The model under review builds one solid part; all positions refer to its coordinate system, in mm. Face numbers are marked on the shaded views. A direction names the side the tool comes from. Give positions to 0.01 mm unless a question says otherwise; leave off trailing zeros. Order: outer loops, then holes, each group sorted by start corner. A loop starts at its lowest first (then second) coordinate and runs counter-clockwise, first axis right, second up. Notation, with made-up numbers: (49, 14.5) - (108, 14.5) arc R29 cw to (108, 51.5) - close; hole circle Ø8 at (12, 40). An arc over 180 degrees is marked (long way). Write item = value, one per line. Start each with the question number.
1. We need section B-B, the plane x = -41.5. Give the boundary of the cut face in (y, z), and give its area (3 significant figures).
2. Wall thickness on probe 1 along Z at (x, y) = (48, -22.5); probe 2 along X at (y, z) = (-19.5, 55); probe 3 along Y at (x, z) = (-24, 51): over which ranges is each line inside the solid? List them lowest first.
3. We need section D-D, the plane x = -1. Give the boundary of the cut face in (y, z), and give its area (3 significant figures).
4. Mouldability with a two-part tool opening along Z and no side actions: class the marked faces 5, 6 and 7 as pulls with the +Z half, pulls with the -Z half, needs draft (parallel to the pull), parting line crosses it, or undercut.
5. For P1, Ø10.5, axis at x = -7, y = -28, coming from the +Z side; P2, Ø4, axis at x = 25, y = 34, coming from the +Z side; P3, Ø12, axis at y = -14.5, z = 24.5, coming from the +X side; P4, Ø8, axis at x = 15.5, z = 73, coming from the -Y side, all flat-tipped, find the tip position at first contact; note any pin that passes through.
6. We need section A-A, the plane y = 0. Give the boundary of the cut face in (x, z).
7. Machinability: for the marked faces 1, 2, 3 and 4, which of the approach directions +Z, -Z, +X, -X, +Y, -Y give a long, thin tool a straight path to every point of the face, cutting with its end or side? Answer none if there is none.
8. We need section C-C, the plane y = 21. Give the boundary of the cut face in (x, z), and give its area (3 significant figures).
from build123d import *

# Parameters (mm, degrees)
F0_W     = 101.6
F0_H     = 48.768
F1_DEPTH = 56.388
F0_H_2   = 13.335
F2_DEPTH = 2.54
F3_R     = 4.7625
F4_DEPTH = 25.4
F3_R_2   = 32.0675
F5_DEPTH = 9.144
F6_DEPTH = 3.81


with BuildPart() as f1:
    # F0 (on Top) → F1 (new body)
    with BuildSketch(Plane.XY):
        Rectangle(F0_W, F0_H)
    extrude(amount=F1_DEPTH)

    # F0 (on Top) → F2 (join)
    with BuildSketch(Plane.XY):
        with Locations((0, 31.0515)):
            Rectangle(F0_W, F0_H_2)
        with Locations((0, -31.0515)):
            Rectangle(F0_W, F0_H_2)
    extrude(amount=F2_DEPTH)

    # F3 (on face) → F4 (join)
    with BuildSketch(Plane.XY.offset(56.388)):
        with Locations((29.21, 0)):
            Circle(F3_R)
    extrude(amount=F4_DEPTH)

    # F3 (on face) → F5 (join)
    with BuildSketch(Plane.XY.offset(56.388)):
        with Locations((29.21, 0)):
            Circle(F3_R_2)
        with Locations((29.21, 0)):
            Circle(F3_R, mode=Mode.SUBTRACT)
    extrude(amount=F5_DEPTH)

    # F3 (on face) → F6 (cut)
    with BuildSketch(Plane.XY.offset(56.388)):
        with Locations((29.21, 0)):
            Circle(F3_R_2)
        with Locations((29.21, 0)):
            Circle(F3_R, mode=Mode.SUBTRACT)
    extrude(amount=F6_DEPTH, mode=Mode.SUBTRACT)


solid = f1.part
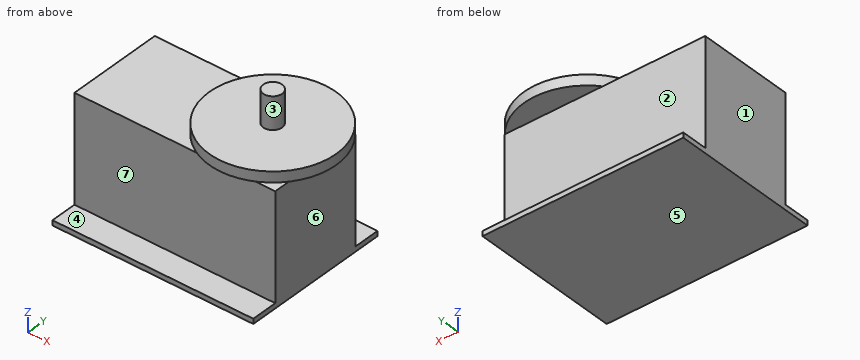
Model answer:
q1.outline = (-37.72, 0) - (37.72, 0) - (37.72, 2.54) - (24.38, 2.54) - (24.38, 56.39) - (-24.38, 56.39) - (-24.38, 2.54) - (-37.72, 2.54) - close
q1.area = 2,820 mm2
q2.probe_1 = 0 to 56.39, 60.2 to 65.53
q2.probe_2 = -50.8 to 50.8
q2.probe_3 = -24.38 to 24.38
q3.outline = (-37.72, 0) - (37.72, 0) - (37.72, 2.54) - (24.38, 2.54) - (24.38, 56.39) - (-24.38, 56.39) - (-24.38, 2.54) - (-37.72, 2.54) - close; (-10.76, 60.2) - (10.76, 60.2) - (10.76, 65.53) - (-10.76, 65.53) - close
q3.area = 2,930 mm2
q4.face_5 = pulls with the -Z half
q4.face_6 = needs draft
q4.face_7 = undercut
q5.P1 = 56.39
q5.P2 = 2.54
q5.P3 = 50.8
q5.P4 = through
q6.outline = (-50.8, 0) - (50.8, 0) - (50.8, 56.39) - (33.97, 56.39) - (33.97, 60.2) - (61.28, 60.2) - (61.28, 65.53) - (33.97, 65.53) - (33.97, 81.79) - (24.45, 81.79) - (24.45, 65.53) - (-2.86, 65.53) - (-2.86, 60.2) - (24.45, 60.2) - (24.45, 56.39) - (-50.8, 56.39) - close
q7.face_1 = +Z, -Z, -X, +Y, -Y
q7.face_2 = +X, -X, +Y
q7.face_3 = +Z
q7.face_4 = +X, -X, -Y
q8.outline = (-50.8, 0) - (50.8, 0) - (50.8, 56.39) - (-50.8, 56.39) - close; (4.98, 60.2) - (53.44, 60.2) - (53.44, 65.53) - (4.98, 65.53) - close
q8.area = 5,990 mm2
